Design review of the part built by this model. Coordinates are the model's own, in mm. Face numbers are marked on the shaded views. A direction names the side the tool comes from. Coordinates: 2 decimals unless noted, no trailing zeros. Loops run counter-clockwise (first coordinate to the right, second up) from the corner with the lowest first, then second, coordinate; pieces in that order, holes last. Notation, with made-up numbers: (42, 73) -> (78, 73) arc R16 cw to (78, 99) -> close; hole circle Ø1 at (23.25, 84.5). An arc over 180 degrees is marked (long way). Answer in a Markdown table with one row per item.
```python
from build123d import *

# Parameters (mm, degrees)
SKETCH1_R                = 44
SKETCH1_R_2              = 2.6
BOSS_EXTRUDE1_DEPTH      = 5
BOSS_EXTRUDE2_START      = -4.5
SKETCH1_3_R              = 44
SKETCH1_3_R_2            = 22.5
BOSS_EXTRUDE2_DEPTH      = 4.5
BOSS_EXTRUDE3_START      = 7.5
SKETCH2_R                = 44
SKETCH2_R_2              = 37.7
BOSS_EXTRUDE3_DEPTH      = 7.5
BOSS_EXTRUDE4_DEPTH      = 6
SKETCH4_R                = 35.25
CUT_EXTRUDE1_DEPTH       = 1
SKETCH5_W                = 4.9
SKETCH5_H                = 40
BOSS_EXTRUDE5_DEPTH      = 20
BOSS_EXTRUDE7_DEPTH      = 1
BOSS_EXTRUDE7_DEPTH_BACK = 1
BOSS_EXTRUDE8_DEPTH      = 1
BOSS_EXTRUDE8_DEPTH_BACK = 1
SKETCH8_R                = 2.6
CUT_EXTRUDE2_DEPTH       = 101.039992003
SKETCH9_R                = 2.6
CUT_EXTRUDE3_DEPTH       = 115.808536268
CUT_EXTRUDE4_DEPTH       = 2.5


with BuildPart() as part:
    # Sketch1 → Boss-Extrude1 (new body)
    with BuildSketch(Plane(origin=(0, 0, 0), x_dir=(0, 0, -1), z_dir=(1, 0, 0))):
        Circle(SKETCH1_R)
        with Locations((4.75, 8.227241336)):
            Circle(SKETCH1_R_2, mode=Mode.SUBTRACT)
        with Locations((9.5, 0)):
            Circle(SKETCH1_R_2, mode=Mode.SUBTRACT)
        with Locations((4.75, -8.227241336)):
            Circle(SKETCH1_R_2, mode=Mode.SUBTRACT)
        with Locations((-4.75, -8.227241336)):
            Circle(SKETCH1_R_2, mode=Mode.SUBTRACT)
        with Locations((-9.5, 0)):
            Circle(SKETCH1_R_2, mode=Mode.SUBTRACT)
        with Locations((-4.75, 8.227241336)):
            Circle(SKETCH1_R_2, mode=Mode.SUBTRACT)
    extrude(amount=BOSS_EXTRUDE1_DEPTH)

    # Sketch1_3 → Boss-Extrude2 (add)
    with BuildSketch(Plane(origin=(0, 0, 0), x_dir=(0, 0, -1), z_dir=(1, 0, 0)).offset(BOSS_EXTRUDE2_START)):
        Circle(SKETCH1_3_R)
        Circle(SKETCH1_3_R_2, mode=Mode.SUBTRACT)
    extrude(amount=BOSS_EXTRUDE2_DEPTH)

    # Sketch2 → Boss-Extrude3 (add)
    with BuildSketch(Plane.ZY.offset(4.5).offset(BOSS_EXTRUDE3_START)):
        Circle(SKETCH2_R)
        Circle(SKETCH2_R_2, mode=Mode.SUBTRACT)
    extrude(amount=-BOSS_EXTRUDE3_DEPTH)

    # Sketch3 → Boss-Extrude4 (add)
    with BuildSketch(Plane.ZY.offset(12)):
        with BuildLine():
            Line((-25, -86), (25, -86))
            Line((25, -86), (25, -36.20773398))
            ThreePointArc((25, -36.20773398), (0, -44), (-25, -36.20773398))
            Line((-25, -36.20773398), (-25, -86))
        make_face()
    extrude(amount=-BOSS_EXTRUDE4_DEPTH)

    # Sketch4 → Cut-Extrude1 (cut)
    with BuildSketch(Plane.ZY.offset(4.5)):
        Circle(SKETCH4_R)
    extrude(amount=-CUT_EXTRUDE1_DEPTH, mode=Mode.SUBTRACT)

    # Sketch5 → Boss-Extrude5 (add)
    with BuildSketch(Plane.ZY.offset(12)):
        with Locations((-22.55, -66)):
            Rectangle(SKETCH5_W, SKETCH5_H)
        Polygon((-25, -41), (-25, -46), (-20.1, -46), (20.1, -46), (25, -46), (25, -41), align=None)
        with Locations((22.55, -66)):
            Rectangle(SKETCH5_W, SKETCH5_H)
    extrude(amount=BOSS_EXTRUDE5_DEPTH)

    # Sketch6 → Boss-Extrude7 (add, two sides: drawn at the far end of the back side and taken through both)
    with BuildSketch(Plane.XY.offset(16.5).offset(-BOSS_EXTRUDE7_DEPTH_BACK)):
        Polygon((5, -40), (-6, -40), (-6, -86), (5, -44), align=None)
    extrude(amount=BOSS_EXTRUDE7_DEPTH + BOSS_EXTRUDE7_DEPTH_BACK)

    # Sketch7 → Boss-Extrude8 (add, two sides: drawn at the far end of the back side and taken through both)
    with BuildSketch(Plane(origin=(0, 0, -16.5), x_dir=(-1, 0, 0), z_dir=(0, 0, -1)).offset(-BOSS_EXTRUDE8_DEPTH_BACK)):
        Polygon((-5, -40), (6, -40), (6, -86), (-5, -44), align=None)
    extrude(amount=BOSS_EXTRUDE8_DEPTH + BOSS_EXTRUDE8_DEPTH_BACK)

    # Sketch8 → Cut-Extrude2 (cut, through all)
    with BuildSketch(Plane(origin=(-6, 0, 0), x_dir=(0, 0, -1), z_dir=(1, 0, 0))):
        with Locations((-10, -76)):
            Circle(SKETCH8_R)
        with Locations((10, -76)):
            Circle(SKETCH8_R)
        with Locations((-10, -56)):
            Circle(SKETCH8_R)
        with Locations((10, -56)):
            Circle(SKETCH8_R)
    extrude(amount=-CUT_EXTRUDE2_DEPTH, mode=Mode.SUBTRACT)

    # Sketch9 → Cut-Extrude3 (cut, through all)
    with BuildSketch(Plane.XY.offset(25)):
        with Locations((-22, -56)):
            Circle(SKETCH9_R)
        with BuildLine():
            ThreePointArc((-24.253333333, -57.297107894), (-24.6, -56), (-24.253333333, -54.702892106))
            Line((-24.253333333, -54.702892106), (-25, -56))
            Line((-25, -56), (-24.253333333, -57.297107894))
        make_face()
        with Locations((-22, -76)):
            Circle(SKETCH9_R)
        with BuildLine():
            ThreePointArc((-24.253333333, -77.297107894), (-24.6, -76), (-24.253333333, -74.702892106))
            Line((-24.253333333, -74.702892106), (-25, -76))
            Line((-25, -76), (-24.253333333, -77.297107894))
        make_face()
    extrude(amount=-CUT_EXTRUDE3_DEPTH, mode=Mode.SUBTRACT)

    # Sketch10 → Cut-Extrude4 (cut)
    with BuildSketch(Plane(origin=(5, 0, 0), x_dir=(0, 0, -1), z_dir=(1, 0, 0))):
        Polygon((9.5, -4.849742261), (13.7, -2.424871131), (13.7, 2.424871131), (9.5, 4.849742261), (5.3, 2.424871131), (5.3, -2.424871131), align=None)
        Polygon((8.95, 5.802370205), (8.95, 10.652112467), (4.75, 13.076983597), (0.55, 10.652112467), (0.55, 5.802370205), (4.75, 3.377499075), align=None)
        Polygon((0.55, -10.652112467), (4.75, -13.076983597), (8.95, -10.652112467), (8.95, -5.802370205), (4.75, -3.377499075), (0.55, -5.802370205), align=None)
        Polygon((-8.95, -5.802370205), (-8.95, -10.652112467), (-4.75, -13.076983597), (-0.55, -10.652112467), (-0.55, -5.802370205), (-4.75, -3.377499075), align=None)
        Polygon((-9.5, 4.849742261), (-13.7, 2.424871131), (-13.7, -2.424871131), (-9.5, -4.849742261), (-5.3, -2.424871131), (-5.3, 2.424871131), align=None)
        Polygon((-0.55, 10.652112467), (-4.75, 13.076983597), (-8.95, 10.652112467), (-8.95, 5.802370205), (-4.75, 3.377499075), (-0.55, 5.802370205), align=None)
    extrude(amount=-CUT_EXTRUDE4_DEPTH, mode=Mode.SUBTRACT)


solid = part.part
```
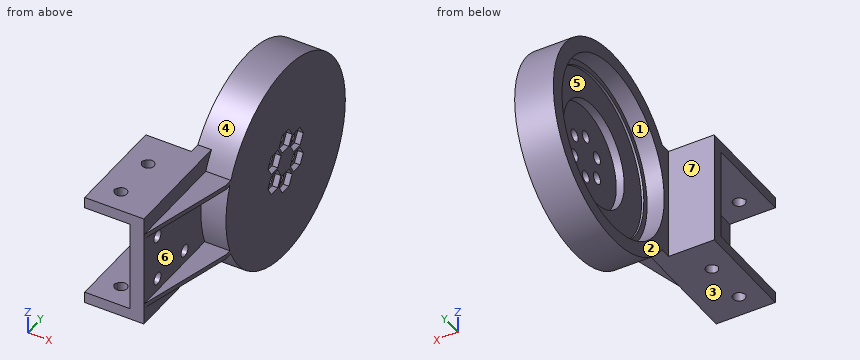
(1) Tool access review of the marked faces 1, 2 and 3: name each direction out of +Z, -Z, +X, -X, +Y, -Y from which nothing blocks a thin tool from reaching the whole face with its end or side.
Evaluation:
| item | result |
|---|---|
| face 1 | -X |
| face 2 | +Z, -Z, -X, +Y |
| face 3 | -Z, +X, -X, -Y |
(2) To check wall thickness, follow probe 1 along Y at (x, z) = (-22, -21.75); probe 2 along Y at (x, z) = (-8, 0); probe 3 along X at (y, z) = (-76, -22.8). State the ranges of each line that lie inside material, in increasing order.
Evaluation:
| item | result |
|---|---|
| probe 1 | y = -86 to -78.6, -73.4 to -58.6, -53.4 to -41 |
| probe 2 | y = -86 to -37.7, 37.7 to 44 |
| probe 3 | x = -32 to -25, -19.4 to -6 |
(3) For pin 1 (2 mm diameter, centred on x = 3.5, y = 9, fed in from -Z); pin 2 (2 mm diameter, centred on y = 11.5, z = 15, fed in from -X); pin 3 (13 mm diameter, centred on x = -17, y = -70, fed in from -Z); pin 4 (4 mm diameter, centred on x = -22, y = -76, fed in from -Z), all flat-tipped, find the tip position at first contact; note any pin that passes through.
Evaluation:
| item | result |
|---|---|
| pin 1 | stops at z = -43.27 |
| pin 2 | stops at x = 0 |
| pin 3 | stops at z = -25 |
| pin 4 | passes through |
(4) Draft analysis for pull direction Y (two halves, no side actions). For the marked faces 4, 5, 6 and 7, state which applies: pulls with the +Y half, pulls with the -Y half, needs draft (parallel to the pull), parting line crosses it, or undercut.
Evaluation:
| item | result |
|---|---|
| face 4 | parting line crosses it |
| face 5 | undercut |
| face 6 | needs draft |
| face 7 | pulls with the +Y half |
(5) Take a section at A-A on x = -22. Give the boundary of the cut face in (y, z).
Evaluation:
| item | result |
|---|---|
| outline | (-86, -25) -> (-78.6, -25) -> (-78.6, -20.1) -> (-86, -20.1) -> close; (-86, 20.1) -> (-78.6, 20.1) -> (-78.6, 25) -> (-86, 25) -> close; (-73.4, -25) -> (-58.6, -25) -> (-58.6, -20.1) -> (-73.4, -20.1) -> close; (-73.4, 20.1) -> (-58.6, 20.1) -> (-58.6, 25) -> (-73.4, 25) -> close; (-53.4, -25) -> (-41, -25) -> (-41, 25) -> (-53.4, 25) -> (-53.4, 20.1) -> (-46, 20.1) -> (-46, -20.1) -> (-53.4, -20.1) -> close |
(6) Take a section at B-B on y = 0. Count the separate pieces of the cut face and the enclosed holes in it, and give its area (4 significant figures).
Evaluation:
| item | result |
|---|---|
| separate pieces | 3 |
| enclosed holes | 0 |
| area | 634.5 mm² |
(7) Take a section at D-D on y = 20.5. Give the boundary of the cut face in (x, z), and give its area (3 significant figures).
Evaluation:
| item | result |
|---|---|
| outline | (-12, -38.93) -> (5, -38.93) -> (5, 38.93) -> (-12, 38.93) -> (-12, 31.64) -> (-4.5, 31.64) -> (-4.5, 28.68) -> (-3.5, 28.68) -> (-3.5, 9.27) -> (0, 9.27) -> (0, -9.27) -> (-3.5, -9.27) -> (-3.5, -28.68) -> (-4.5, -28.68) -> (-4.5, -31.64) -> (-12, -31.64) -> close |
| area | 727 mm² |
(8) Take a section at C-C on z = -28.5. Give the boundary of the cut face in (x, y).
Evaluation:
| item | result |
|---|---|
| outline | (-12, -33.52) -> (5, -33.52) -> (5, 33.52) -> (-12, 33.52) -> (-12, 24.68) -> (-4.5, 24.68) -> (-4.5, 20.74) -> (-3.5, 20.74) -> (-3.5, -20.74) -> (-4.5, -20.74) -> (-4.5, -24.68) -> (-12, -24.68) -> close |
